The listing builds one solid part. Answer for the finished solid, in the listing's coordinates (mm). Face numbers are marked on the shaded views. Coordinates: 2 decimals unless noted, no trailing zeros. Loops run counter-clockwise (first coordinate to the right, second up) from the corner with the lowest first, then second, coordinate; pieces in that order, holes last. Notation, with made-up numbers: M -30.75,-19 L 26.25,-19 A27 ccw 26.25,5 Z; hole C 70,51.5 d3. An arc over 180 degrees is marked long. Answer as a JSON object with one key per item and string values. Group by question number.
1. A cutting plane is placed at A-A on z = 51. Give the vertices of the cut face in (x, y).
2. A cutting plane is placed at B-B on z = 68. Give the vertices of the cut face in (x, y).
3. Determine the mould class of the marked faces 1, 2 and 3 for opening direction Y: released by +Y, released by -Y, zero draft, split by the parting line, or undercut.
4. Given pin 1 (1.5 mm diameter, centred on x = 1, z = 25, fed in from -Y); pin 2 (1 mm diameter, centred on x = -6.5, z = 39.5, fed in from -Y); pin 3 (11 mm diameter, centred on x = -10.42, y = 0, fed in from +Z), each flat-ended and moving along its own axis, determine where each tip first touches the part or whether it passes through.
5. Straight lines are drawn through the part: L1, parallel to Z at x = 3, y = -28; L2, parallel to Y at x = -3, z = 66.5; L3, parallel to Y at x = -2.5, z = 69.5. For each, find the intervals that lie inside material, in ascending order.
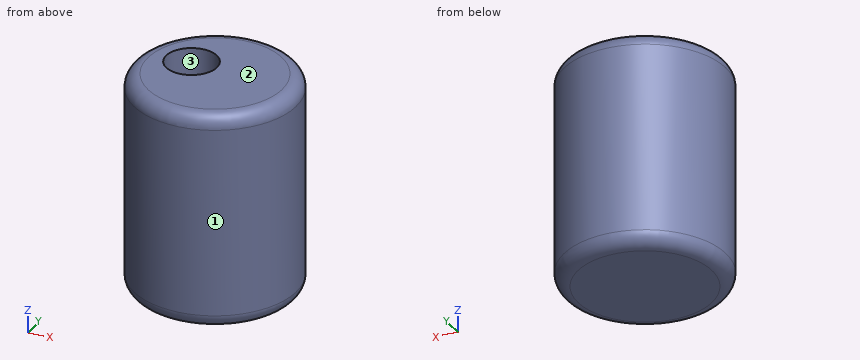
from build123d import *

# Parameters (mm, degrees)
F0_R     = 29.083319
F1_DEPTH = 77.7
F2_R     = 9.110052
F3_DEPTH = 25
F4_R     = 5


with BuildPart() as f1:
    # F0 (on Top) → F1 (new body)
    with BuildSketch(Plane.XY):
        with Locations((0, -3.755013)):
            Circle(F0_R)
    extrude(amount=F1_DEPTH)

    # F2 (on face) → F3 (cut)
    with BuildSketch(Plane.XY.offset(77.7)):
        with Locations((-10.418282, 0)):
            Circle(F2_R)
    extrude(amount=-F3_DEPTH, mode=Mode.SUBTRACT)

    # F4
    f4_edges = [f1.edges().sort_by_distance(p)[0] for p in [
        (-29.083319, -3.755013, 77.7),
        (-29.083319, -3.755013, 0),
    ]]
    fillet(f4_edges, radius=F4_R)


solid = f1.part
From the geometry:
{
 "1": {"outline": "C 0,-3.76 d58.17"},
 "2": {"outline": "C 0,-3.76 d58.17; hole C -10.42,0 d18.22"},
 "3": {"face 1": "split by the parting line", "face 2": "zero draft", "face 3": "undercut"},
 "4": {"pin 1": "stops at y = -32.84", "pin 2": "stops at y = -32.21", "pin 3": "stops at z = 52.7"},
 "5": {"L1": "z = 0.01 to 77.69", "L2": "y = -32.68 to -5.29, 5.29 to 25.17", "L3": "y = -32.73 to -4.5, 4.5 to 25.22"}
}
